Input: part model. Units: mm. Frame: model coordinates. A direction names the side the tool comes from. Give positions to 0.01 mm unless a question says otherwise; leave off trailing zeros. Order: outer loops, then holes, each group sorted by start corner. A loop starts at its lowest first (then second) coordinate and runs counter-clockwise, first axis right, second up. Notation, with made-up numbers: (-15.5, -19) - (-4.5, -19) arc R10 ccw to (-4.5, -11) - close; hole circle Ø7 at (50.25, 79.5). An arc over 180 degrees is marked (long way). Use a Markdown table: item, result.
from build123d import *

# Parameters (mm, degrees)
SKETCH1_W           = 16
SKETCH1_H           = 16
BOSS_EXTRUDE1_DEPTH = 3.2
SKETCH2_R           = 2.4
BOSS_EXTRUDE2_DEPTH = 1.8
SKETCH3_W           = 12.8
SKETCH3_H           = 12.8
CUT_EXTRUDE1_DEPTH  = 1.8
SKETCH4_R           = 3.25685425
BOSS_EXTRUDE3_DEPTH = 1.8
SKETCH5_R           = 2.45685425
CUT_EXTRUDE2_DEPTH  = 1.8


with BuildPart() as part:
    # Sketch1 → Boss-Extrude1 (new body)
    with BuildSketch(Plane(origin=(0, 0, 0), x_dir=(1, 0, 0), z_dir=(0, 1, 0))):
        with Locations((8, 8)):
            Rectangle(SKETCH1_W, SKETCH1_H)
    extrude(amount=BOSS_EXTRUDE1_DEPTH)

    # Sketch2 → Boss-Extrude2 (add)
    with BuildSketch(Plane(origin=(0, 3.2, 0), x_dir=(1, 0, 0), z_dir=(0, 1, 0))):
        with Locations(Location((4, 12, 0), (0, 0, 90))):
            Circle(SKETCH2_R)
        with Locations(Location((12, 12, 0), (0, 0, 90))):
            Circle(SKETCH2_R)
        with Locations(Location((12, 4, 0), (0, 0, 90))):
            Circle(SKETCH2_R)
        with Locations(Location((4, 4, 0), (0, 0, 90))):
            Circle(SKETCH2_R)
    extrude(amount=BOSS_EXTRUDE2_DEPTH)

    # Sketch3 → Cut-Extrude1 (cut)
    with BuildSketch(Plane.XZ):
        with Locations((8, -8)):
            Rectangle(SKETCH3_W, SKETCH3_H)
    extrude(amount=-CUT_EXTRUDE1_DEPTH, mode=Mode.SUBTRACT)

    # Sketch4 → Boss-Extrude3 (add)
    with BuildSketch(Plane.XZ.offset(-1.8)):
        with Locations(Location((8, -8, 0), (0, 0, 270))):
            Circle(SKETCH4_R)
    extrude(amount=BOSS_EXTRUDE3_DEPTH)

    # Sketch5 → Cut-Extrude2 (cut)
    with BuildSketch(Plane.XZ):
        with Locations(Location((8, -8, 0), (0, 0, 270))):
            Circle(SKETCH5_R)
    extrude(amount=-CUT_EXTRUDE2_DEPTH, mode=Mode.SUBTRACT)


solid = part.part
1. Mould query, pull axis X, two halves, no side actions, for faces 1 (the face through (4, 5, -12)), 2 (the face through (3.28, 4.09, -6.29)), 3 (the face through (0, 2, -8)). Classes: pulls with the +X half, pulls with the -X half, needs draft (parallel to the pull), parting line crosses it, or undercut.
Response:
| item | result |
|---|---|
| face 1 | needs draft |
| face 2 | undercut |
| face 3 | pulls with the -X half |
2. Section query B-B (z = -4). Return loops of the section in (x, y), then the cut area to 3 significant figures.
Response:
| item | result |
|---|---|
| outline | (0, 0) - (1.6, 0) - (1.6, 1.8) - (14.4, 1.8) - (14.4, 0) - (16, 0) - (16, 3.2) - (14.4, 3.2) - (14.4, 5) - (9.6, 5) - (9.6, 3.2) - (6.4, 3.2) - (6.4, 5) - (1.6, 5) - (1.6, 3.2) - (0, 3.2) - close |
| area | 45.4 mm^2 |
3. Set-up query: faces 4 (the face through (15, 0, -8)), 5 (the face through (9.62, 4.09, -11.69)), 6 (the face through (10.746, 0.913, -9.751)). Return all of +Z, -Z, +X, -X, +Y, -Y with unobstructed straight access to the full face (end or side cutting, diameter ignored); none if empty.
Response:
| item | result |
|---|---|
| face 4 | +Z, -Z, +X, -X, -Y |
| face 5 | +Y |
| face 6 | -Y |
4. Section query C-C (x = 12). Return loops of the section in (y, z), then the cut area to 3 significant figures.
Response:
| item | result |
|---|---|
| outline | (0, -16) - (3.2, -16) - (3.2, -14.4) - (5, -14.4) - (5, -9.6) - (3.2, -9.6) - (3.2, -6.4) - (5, -6.4) - (5, -1.6) - (3.2, -1.6) - (3.2, 0) - (0, 0) - (0, -1.6) - (1.8, -1.6) - (1.8, -14.4) - (0, -14.4) - close |
| area | 45.4 mm^2 |
5. Section query A-A (y = 1.1). Return loops of the section in (x, z).
Response:
| item | result |
|---|---|
| outline | (0, -16) - (16, -16) - (16, 0) - (0, 0) - close; circle Ø6.51 at (8, -8); hole (1.6, -14.4) - (14.4, -14.4) - (14.4, -1.6) - (1.6, -1.6) - close; hole circle Ø4.91 at (8, -8) |
6. Pin query (flat end, axial travel): pin 1 (1.5 mm diameter, centred on x = 8.5, y = 0.5, fed in from +Z); pin 2 (4.5 mm diameter, centred on x = 8, z = -8, fed in from +Y); pin 3 (1.5 mm diameter, centred on x = 7.5, z = -8, fed in from -Y). Return the tip coordinate at first contact, or that it passes through.
Response:
| item | result |
|---|---|
| pin 1 | stops at z = 0 |
| pin 2 | stops at y = 3.2 |
| pin 3 | stops at y = 1.8 |
7. Material intervals for line 1 along X through (y, z) = (0.7, -8); line 2 along X through (y, z) = (0.6, -9.5); line 3 along X through (y, z) = (1.7, -13.25), sorted ascending.
Response:
| item | result |
|---|---|
| line 1 | x = 0 to 1.6, 4.74 to 5.54, 10.46 to 11.26, 14.4 to 16 |
| line 2 | x = 0 to 1.6, 5.11 to 6.05, 9.95 to 10.89, 14.4 to 16 |
| line 3 | x = 0 to 1.6, 14.4 to 16 |
